CAD build for the part. Positions are in the model's coordinates, mm. A direction names the side the tool comes from. Round coordinates to 2 decimals unless told otherwise and drop trailing zeros. Order: outer loops, then holes, each group sorted by start corner. A loop starts at its lowest first (then second) coordinate and runs counter-clockwise, first axis right, second up. Notation, with made-up numbers: (-21.5, 35) -> (7.5, 35) arc R15 cw to (7.5, 60) -> close; hole circle Ø8 at (12.5, -4.5). An arc over 180 degrees is marked (long way). Return JSON: item names as keys, results as strings. Group by question number.
Q1. Flat gauge pins, fed straight in: pin 1 (4.5 mm diameter, centred on x = 39.5, y = 1, fed in from +Z); pin 2 (1 mm diameter, centred on x = 17, y = 11, fed in from +Z); pin 3 (4.5 mm diameter, centred on x = 25, z = 7, fed in from -Y). Where does each tip first touch, or does it go through?
Q2. Mould opens along Y. For faces 6 (the flat face through (20.2, 0, 1.5)), 7 (the flat face through (39, 4, 6)), 8 (the flat face through (9.362, 39, -3)) say: +Y half, -Y half, draft (parallel to the pull), parting line (faces both ways), or undercut.
Q3. Probe line 1 along Y through (x, z) = (36.5, 7.5); line 2 along Y through (x, z) = (3.5, 7.25); line 3 along Z through (x, y) = (31, 33.5). List the from-to ranges inside material, lowest first.
Q4. Cut at A-A (y = 34). Write the cut outline in (x, z), then the cut area to 3 significant figures.
Q5. Cut at D-D (y = 19). Write the cut outline in (x, z).
Q6. Which spindle directions (+Z, -Z, +X, -X, +Y, -Y) get a long thin tool onto all of the face, cutting with end or side? Do faces 1 (the flat face through (9, 32, -3)), 2 (the flat face through (2, 4, 6)), 3 (the flat face through (7.862, 39, -3)), 4 (the flat face through (6.316, 21, 1)), 5 (the flat face through (37, 2, 6)). Say none if no direction does.
Q7. Cut at B-B (z = 6.25). Write the cut outline in (x, y), then the cut area to 3 significant figures.
Q8. Cut at C-C (x = 5). Write the cut outline in (y, z), then the cut area to 3 significant figures.
from build123d import *

# Parameters (mm, degrees)
SCHIZZO1_W                   = 41
SCHIZZO1_H                   = 46
ESTRUSIONE_ESTRUSIONE1_DEPTH = 2
SCHIZZO2_W                   = 4
SCHIZZO2_H                   = 4
ESTRUSIONE_ESTRUSIONE2_DEPTH = 7.5
SCHIZZO3_W                   = 41
SCHIZZO3_H                   = 3.7
ESTRUSIONE_ESTRUSIONE3_DEPTH = 15.6
SCHIZZO4_W                   = 6.315683346
SCHIZZO4_H                   = 34.34145986
TAGLIO_ESTRUSIONE1_DEPTH     = 2
SCHIZZO5_W                   = 1.5
SCHIZZO5_H                   = 14
ESTRUSIONE_ESTRUSIONE4_DEPTH = 6
SCHIZZO7_R                   = 5.421973109
TAGLIO_ESTRUSIONE3_DEPTH     = 2


with BuildPart() as part:
    # Schizzo1 → Estrusione-Estrusione1 (new body)
    with BuildSketch(Plane.XY):
        with Locations((20.5, 23)):
            Rectangle(SCHIZZO1_W, SCHIZZO1_H)
    extrude(amount=ESTRUSIONE_ESTRUSIONE1_DEPTH)

    # Schizzo2 → Estrusione-Estrusione2 (add)
    with BuildSketch(Plane.XY.offset(2)):
        with Locations((2, 2)):
            Rectangle(SCHIZZO2_W, SCHIZZO2_H)
        with Locations((39, 2)):
            Rectangle(SCHIZZO2_W, SCHIZZO2_H)
    extrude(amount=ESTRUSIONE_ESTRUSIONE2_DEPTH)

    # Schizzo3 → Estrusione-Estrusione3 (add)
    with BuildSketch(Plane.XY.offset(2)):
        with Locations((20.5, 44.15)):
            Rectangle(SCHIZZO3_W, SCHIZZO3_H)
    extrude(amount=ESTRUSIONE_ESTRUSIONE3_DEPTH)

    # Schizzo4 → Taglio-Estrusione1 (cut)
    with BuildSketch(Plane(origin=(0, 0, 0), x_dir=(-1, 0, 0), z_dir=(0, 0, -1))):
        with Locations((-3.157841673, 21.578763697)):
            Rectangle(SCHIZZO4_W, SCHIZZO4_H)
    extrude(amount=-TAGLIO_ESTRUSIONE1_DEPTH, mode=Mode.SUBTRACT)

    # Schizzo5 → Estrusione-Estrusione4 (add)
    with BuildSketch(Plane(origin=(0, 0, 0), x_dir=(-1, 0, 0), z_dir=(0, 0, -1))):
        with Locations((-8.611501058, 39)):
            Rectangle(SCHIZZO5_W, SCHIZZO5_H)
    extrude(amount=ESTRUSIONE_ESTRUSIONE4_DEPTH)

    # Schizzo7 → Taglio-Estrusione3 (cut)
    with BuildSketch(Plane(origin=(0, 0, 0), x_dir=(-1, 0, 0), z_dir=(0, 0, -1))):
        with Locations((-23.8073986, 23.20549075)):
            Circle(SCHIZZO7_R)
    extrude(amount=-TAGLIO_ESTRUSIONE3_DEPTH, mode=Mode.SUBTRACT)


solid = part.part
Solution:
{
 "1": {"pin 1": "stops at z = 9.5", "pin 2": "stops at z = 2", "pin 3": "stops at y = 42.3"},
 "2": {"face 6": "-Y half", "face 7": "undercut", "face 8": "draft"},
 "3": {"line 1": "y = 42.3 to 46", "line 2": "y = 0 to 4, 42.3 to 46", "line 3": "z = 0 to 2"},
 "4": {"outline": "(6.32, 0) -> (7.86, 0) -> (7.86, -6) -> (9.36, -6) -> (9.36, 0) -> (41, 0) -> (41, 2) -> (6.32, 2) -> close", "area": "78.4 mm²"},
 "5": {"outline": "(6.32, 0) -> (20.39, 0) -> (20.39, 2) -> (6.32, 2) -> close; (27.23, 0) -> (41, 0) -> (41, 2) -> (27.23, 2) -> close"},
 "6": {"face 1": "-Z, +X, -X, -Y", "face 2": "+Z, +X, -X", "face 3": "-Z, -X, +Y, -Y", "face 4": "+Z, -Z, -X", "face 5": "+Z, -Y"},
 "7": {"outline": "(0, 0) -> (4, 0) -> (4, 4) -> (0, 4) -> close; (0, 42.3) -> (41, 42.3) -> (41, 46) -> (0, 46) -> close; (37, 0) -> (41, 0) -> (41, 4) -> (37, 4) -> close", "area": "184 mm²"},
 "8": {"outline": "(0, 0) -> (4.41, 0) -> (4.41, 2) -> (0, 2) -> close; (38.75, 0) -> (46, 0) -> (46, 17.6) -> (42.3, 17.6) -> (42.3, 2) -> (38.75, 2) -> close", "area": "81.0 mm²"}
}
